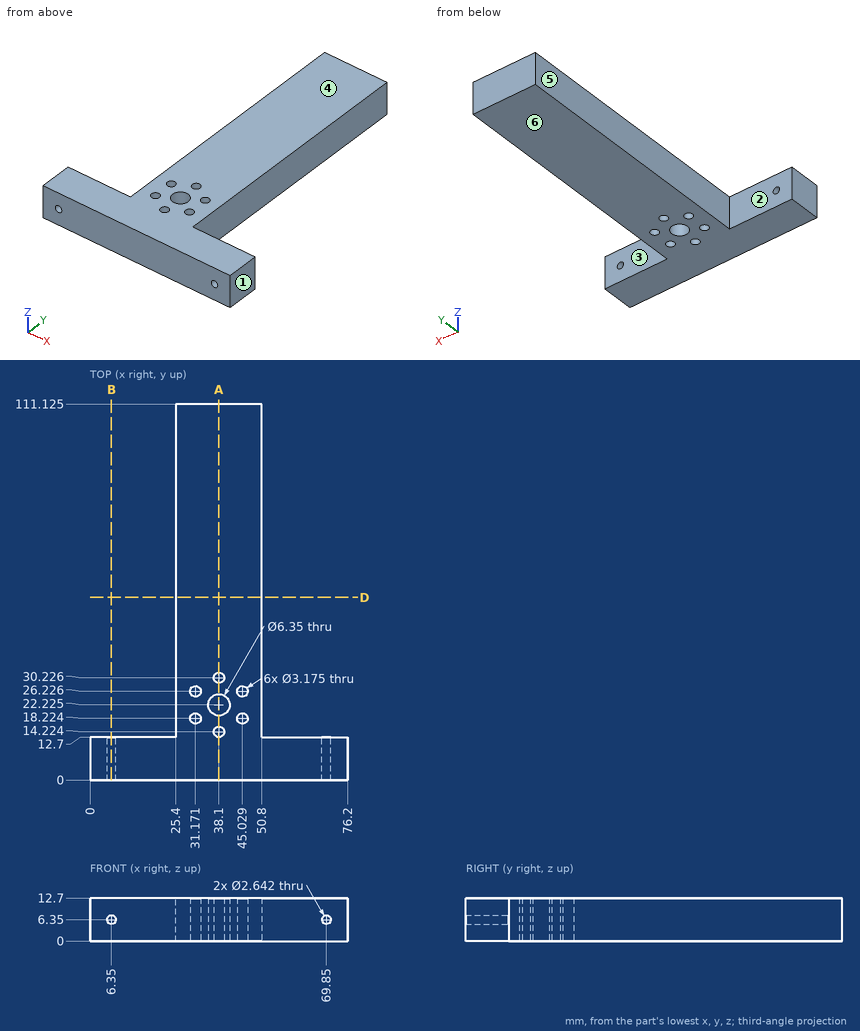
Job drawing, mm, ordinate dimensions from the low corner. One solid piece. A direction names the side the tool comes from. Give positions to 0.01 mm unless a question says otherwise; leave off trailing zeros. Order: outer loops, then holes, each group sorted by start corner. A loop starts at its lowest first (then second) coordinate and runs counter-clockwise, first axis right, second up. Notation, with made-up numbers: (-28.75, -22) - (-22.75, -22) arc R22 ccw to (-22.75, -11) - close; hole circle Ø10 at (-28.75, 34). An arc over 180 degrees is marked (long way). One line per question, with ' | ' between items.
1. Band-saw the part on B-B on x = 6.35. List the corners of the cut face in (y, z).
Filled in:
outline: (0, 0) - (12.7, 0) - (12.7, 5.03) - (0, 5.03) - close; (0, 7.67) - (12.7, 7.67) - (12.7, 12.7) - (0, 12.7) - close
2. Drill centre lines: probe 1 along X at (y, z) = (9.5, 6.35); probe 2 along X at (y, z) = (19.5, 7.75) (1 decimal); probe 3 along Z at (x, y) = (6.35, 4.25). Where is each one in solid material? Low to high.
Filled in:
probe 1: 0 to 5.03, 7.67 to 68.53, 71.17 to 76.2 | probe 2: 25.4 to 30.2, 32.1 to 36.5, 39.7 to 44.1, 46 to 50.8 | probe 3: 0 to 5.03, 7.67 to 12.7
3. Which spindle directions (+Z, -Z, +X, -X, +Y, -Y) get a long thin tool onto all of the face, cutting with end or side? Do the marked faces 1, 2 and 3. Say none if no direction does.
Filled in:
face 1: +Z, -Z, +X, +Y, -Y | face 2: +Z, -Z, -X, +Y | face 3: +Z, -Z, +X, +Y
4. Pull direction Z, two halves, no side cores. Call the marked faces 4, 5 and 6: +Z half, -Z half, draft (parallel to the pull), parting line (faces both ways), or undercut.
Filled in:
face 4: +Z half | face 5: draft | face 6: -Z half
5. Band-saw the part on A-A on x = 38.1. Give the number of separate pieces and of enclosed holes in the cut face, then the cut area to 3 significant figures.
Filled in:
separate pieces: 4 | enclosed holes: 0 | area: 1,250 mm²
6. Drop flat-ended pins along their axis: P1, Ø4, axis at x = 8, z = 3.5, coming from the +Y side; P2, Ø6, axis at y = 37.5, z = 7.5, coming from the -X side; P3, Ø3, axis at y = 40.5, z = 10, coming from the +X side. Give the stop position or say it passes through.
Filled in:
P1: y = 12.7 | P2: x = 25.4 | P3: x = 50.8
7. Band-saw the part on D-D on y = 54. List the corners of the cut face in (x, z), then the cut area to 3 significant figures.
Filled in:
outline: (25.4, 0) - (50.8, 0) - (50.8, 12.7) - (25.4, 12.7) - close | area: 323 mm²
